The listing builds one solid part. Answer for the finished solid, in the listing's coordinates (mm). Face numbers are marked on the shaded views. A direction names the side the tool comes from. Coordinates: 2 decimals unless noted, no trailing zeros. Order: outer loops, then holes, each group sorted by start corner. A loop starts at its lowest first (then second) coordinate and runs counter-clockwise, first axis right, second up. Notation, with made-up numbers: M -4,-25.5 L 4,-25.5 A21 cw 4,-14.5 Z; hole C 71.25,-2 d9. An arc over 180 degrees is marked long. One line per item, written item: value. Start each with the question number.
Q1. The part is cut by section C-C on z = 4. Give the vertices of the cut face in (x, y) (3 decimals), then the cut area to 3 significant figures.
Q2. Determine the mould class of the marked faces 1, 2 and 3 for opening direction Y: pulls with the +Y half, pulls with the -Y half, needs draft (parallel to the pull), parting line crosses it, or undercut.
Q3. Straight lines are drawn through the part: line 1 along Y through (x, z) = (0, 8.25) (3 decimals); line 2 along Y through (x, z) = (0, -0.75) (3 decimals); line 3 along X through (y, z) = (0.5, 5.75) (3 decimals). For each, find the intervals that lie inside material, in ascending order. Write a range as [from, to].
Q4. The part is cut by section A-A on x = 0. Give the vertices of the cut face in (y, z) (3 decimals).
Q5. The part is cut by section D-D on z = 13. Give the vertices of the cut face in (x, y), then the cut area to 3 significant figures.
Q6. For the marked faces 4 and 5, determine the directions among +Z, -Z, +X, -X, +Y, -Y from which every point of the face is accessible in a straight line to the end or side of a thin tool.
Q7. Each of these flat-tipped pins is pushed along its axis until it touches: pin 1 Ø4 at (y, z) = (-9.5, 1.5) entering from -X; pin 2 Ø2.5 at (x, y) = (0, -9.315) entering from +Z; pin 3 Ø1 at (x, z) = (-4.5, 12.5) entering from +Y; pin 4 Ø10 at (x, z) = (6.5, 0) entering from +Y. Where does it stop, or does it pass through?
```python
from build123d import *

# Parameters (mm, degrees)
SKETCH1_R           = 12.5
BOSS_EXTRUDE1_DEPTH = 7.5
CUT_EXTRUDE1_REACH  = 25.184
SKETCH8_W           = 12.25
SKETCH8_H           = 12.25
SKETCH11_R          = 1.45
CUT_EXTRUDE4_DEPTH  = 24.184046239
BOSS_EXTRUDE2_START = 5
SKETCH14_R          = 12.5
BOSS_EXTRUDE2_DEPTH = 5
SKETCH15_R          = 3.95
BOSS_EXTRUDE3_DEPTH = 7
CHAMFER1_SIZE       = 0.5
SKETCH18_R          = 1.45
CUT_EXTRUDE6_DEPTH  = 30


with BuildPart() as part:
    # Sketch1 → Boss-Extrude1 (new, symmetric)
    with BuildSketch(Plane.XY):
        Circle(SKETCH1_R)
    extrude(amount=BOSS_EXTRUDE1_DEPTH, both=True)

    # Sketch8 → Cut-Extrude1 (cut, up to next)
    with BuildSketch(Plane.XY.offset(7.5), mode=Mode.PRIVATE) as cut_extrude1_sk1:
        Rectangle(SKETCH8_W, SKETCH8_H)
    cut_extrude1_tool1 = extrude(cut_extrude1_sk1.sketch, amount=-CUT_EXTRUDE1_REACH, mode=Mode.PRIVATE) & part.part
    add(cut_extrude1_tool1.solids().sort_by_distance((0, 0, 7.5))[0], mode=Mode.SUBTRACT)

    # Sketch11 → Cut-Extrude4 (cut, through all)
    with BuildSketch(Plane.XY.offset(7.5)):
        with Locations((9.315, 0)):
            Circle(SKETCH11_R)
        with Locations((0, -9.315)):
            Circle(SKETCH11_R)
        with Locations((-9.315, 0)):
            Circle(SKETCH11_R)
        with Locations((0, 9.315)):
            Circle(SKETCH11_R)
    extrude(amount=-CUT_EXTRUDE4_DEPTH, mode=Mode.SUBTRACT)

    # Sketch14 → Boss-Extrude2 (add)
    with BuildSketch(Plane.XY.offset(7.5).offset(BOSS_EXTRUDE2_START)):
        Circle(SKETCH14_R)
    extrude(amount=-BOSS_EXTRUDE2_DEPTH)

    # Sketch13 → Revolve1 (revolve)
    with BuildSketch(Plane(origin=(0, 0, 0), x_dir=(1, 0, 0), z_dir=(0, 1, 0)), mode=Mode.PRIVATE) as revolve1_sk:
        Polygon((0, -15.5), (3.95, -15.5), (7.5, -8.506732209), (0, -8.506732209), align=None)
    revolve(revolve1_sk.sketch.rotate(Axis((0, 0, 11.965062333), (0, 0, 1)), 180), axis=Axis((0, 0, 11.965062333), (0, 0, 1)))

    # Sketch15 → Boss-Extrude3 (add)
    with BuildSketch(Plane.XY.offset(15.5)):
        Circle(SKETCH15_R)
    extrude(amount=BOSS_EXTRUDE3_DEPTH)

    # Chamfer1
    chamfer1_edges = [part.edges().sort_by_distance(p)[0] for p in [
        (-3.95, 0, 22.5),
    ]]
    chamfer(chamfer1_edges, length=CHAMFER1_SIZE)

    # Sketch18 → Cut-Extrude6 (cut)
    with BuildSketch(Plane.XY.offset(12.5)):
        with Locations((-9.315, 0)):
            Circle(SKETCH18_R)
        with Locations((0, -9.315)):
            Circle(SKETCH18_R)
        with Locations((9.315, 0)):
            Circle(SKETCH18_R)
        with Locations((0, 9.315)):
            Circle(SKETCH18_R)
    extrude(amount=-CUT_EXTRUDE6_DEPTH, mode=Mode.SUBTRACT)


solid = part.part
```
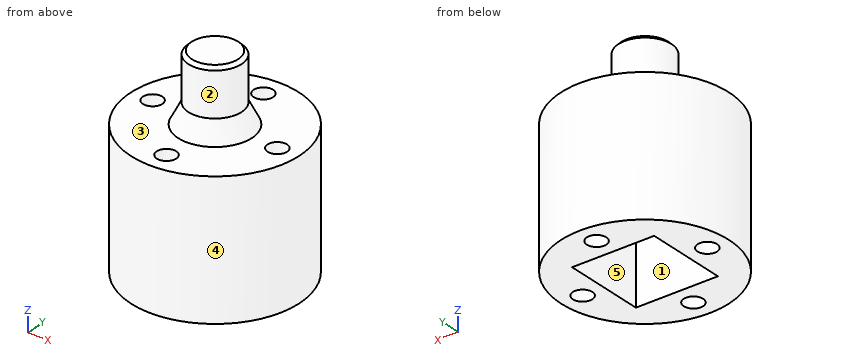
Output:
1. outline: C 0,0 d25; hole C -9.315,0 d2.9; hole M -6.125,-6.125 L 6.125,-6.125 L 6.125,6.125 L -6.125,6.125 Z; hole C 0,-9.315 d2.9; hole C 0,9.315 d2.9; hole C 9.315,0 d2.9
1. area: 314 mm^2
2. face 1: undercut
2. face 2: parting line crosses it
2. face 3: needs draft
3. line 1: y = [-12.5, -10.765], [-7.865, 7.865], [10.765, 12.5]
3. line 2: y = [-12.5, -10.765], [-7.865, -6.125], [6.125, 7.865], [10.765, 12.5]
3. line 3: x = [-12.49, -10.676], [-7.954, -6.125], [6.125, 7.954], [10.676, 12.49]
4. outline: M -12.5,-7.5 L -10.765,-7.5 L -10.765,12.5 L -12.5,12.5 Z; M -7.865,-7.5 L -6.125,-7.5 L -6.125,7.5 L 6.125,7.5 L 6.125,-7.5 L 7.865,-7.5 L 7.865,12.5 L 5.473,12.5 L 3.95,15.5 L 3.95,22 L 3.45,22.5 L -3.45,22.5 L -3.95,22 L -3.95,15.5 L -5.473,12.5 L -7.865,12.5 Z; M 10.765,-7.5 L 12.5,-7.5 L 12.5,12.5 L 10.765,12.5 Z
5. outline: C 0,0 d10.44
5. area: 85.6 mm^2
6. face 4: +Z, -Z
6. face 5: -Z
7. pin 1: stops at x = -10
7. pin 2: passes through
7. pin 3: stops at y = 11.84
7. pin 4: stops at y = 12.41
